from build123d import *

# Parameters (mm, degrees)
CROQUIS1_W              = 471.25
CROQUIS1_H              = 55
SALIENTE_EXTRUIR1_DEPTH = 4
CROQUIS2_W              = 471.25
CROQUIS2_H              = 4
SALIENTE_EXTRUIR2_DEPTH = 55
REDONDEO1_R             = 3
REDONDEO2_R             = 1.5
CORTAR_EXTRUIR1_REACH   = 246.451
CROQUIS3_R              = 2


with BuildPart() as part:
    # Croquis1 → Saliente-Extruir1 (new body)
    with BuildSketch(Plane.XY):
        Rectangle(CROQUIS1_W, CROQUIS1_H)
    extrude(amount=SALIENTE_EXTRUIR1_DEPTH)

    # Croquis2 → Saliente-Extruir2 (add)
    with BuildSketch(Plane(origin=(0, 0, 0), x_dir=(-1, 0, 0), z_dir=(0, 0, -1))):
        with Locations((0, -25.5)):
            Rectangle(CROQUIS2_W, CROQUIS2_H)
    extrude(amount=SALIENTE_EXTRUIR2_DEPTH)

    # Redondeo1
    redondeo1_edges = [part.edges().sort_by_distance(p)[0] for p in [
        (0, -23.5, 0),
    ]]
    fillet(redondeo1_edges, radius=REDONDEO1_R)

    # Redondeo2
    redondeo2_edges = [part.edges().sort_by_distance(p)[0] for p in [
        (0, -27.5, 4),
    ]]
    fillet(redondeo2_edges, radius=REDONDEO2_R)

    # Croquis3 → Cortar-Extruir1 (cut, up to next)
    with BuildSketch(Plane.XY.offset(4), mode=Mode.PRIVATE) as cortar_extruir1_sk1:
        with Locations((-115, -11.2375)):
            Circle(CROQUIS3_R)
    cortar_extruir1_tool1 = extrude(cortar_extruir1_sk1.sketch, amount=-CORTAR_EXTRUIR1_REACH, mode=Mode.PRIVATE) & part.part
    # Croquis3 → Cortar-Extruir1 (cut, up to next)
    with BuildSketch(Plane.XY.offset(4), mode=Mode.PRIVATE) as cortar_extruir1_sk2:
        with Locations((0, -11.2375)):
            Circle(CROQUIS3_R)
    cortar_extruir1_tool2 = extrude(cortar_extruir1_sk2.sketch, amount=-CORTAR_EXTRUIR1_REACH, mode=Mode.PRIVATE) & part.part
    # Croquis3 → Cortar-Extruir1 (cut, up to next)
    with BuildSketch(Plane.XY.offset(4), mode=Mode.PRIVATE) as cortar_extruir1_sk3:
        with Locations((115, -11.2375)):
            Circle(CROQUIS3_R)
    cortar_extruir1_tool3 = extrude(cortar_extruir1_sk3.sketch, amount=-CORTAR_EXTRUIR1_REACH, mode=Mode.PRIVATE) & part.part
    add(cortar_extruir1_tool1.solids().sort_by_distance((-115, -11.2375, 4))[0], mode=Mode.SUBTRACT)
    add(cortar_extruir1_tool2.solids().sort_by_distance((0, -11.2375, 4))[0], mode=Mode.SUBTRACT)
    add(cortar_extruir1_tool3.solids().sort_by_distance((115, -11.2375, 4))[0], mode=Mode.SUBTRACT)


solid = part.part
Could you check a few things on this model? Use its own coordinates, in mm. A direction names the side the tool comes from. Round coordinates to 2 decimals unless told otherwise and drop trailing zeros. Order: outer loops, then holes, each group sorted by start corner. A loop starts at its lowest first (then second) coordinate and runs counter-clockwise, first axis right, second up. Notation, with made-up numbers: M 48,-16.5 L 94,-16.5 A23 ccw 94,17.5 Z; hole C 67,43 d3. An arc over 180 degrees is marked long. One line per item, written item: value.
(1) Imagine slicing it at B-B (y = 21.5). Write out the boundary of the cut face in (x, z) (3 decimals), and give its area (4 significant figures).
Ans:
outline: M -235.625,0 L 235.625,0 L 235.625,4 L -235.625,4 Z
area: 1,885 mm^2
(2) Which directions (+Z, -Z, +X, -X, +Y, -Y) give clear straight access to the entire face, cutting with the end or side of a thin tool? Please do faces 1 (the flat face through (-235.625, -25, -12)), 2 (the flat face through (3, -23.5, -29)).
Ans:
face 1: +Z, -Z, -X, +Y, -Y
face 2: -Z, +X, -X, +Y
(3) Imagine slicing it at C-C (z = -51). Write out the boundary of the cut face in (x, y) (3 decimals), and give its area (4 significant figures).
Ans:
outline: M -235.625,-27.5 L 235.625,-27.5 L 235.625,-23.5 L -235.625,-23.5 Z
area: 1,885 mm^2
(4) I need wall thicknesses on line 1 along Y through (x, z) = (115, 0.8); line 2 along Z through (x, y) = (212.5, -12); line 3 along Y through (x, z) = (151, -50.5). Which ranges of each line are inside material? Lowest first, please. Write a range as from..to.
Ans:
line 1: y = -27.5..-13.24, -9.24..27.5
line 2: z = 0..4
line 3: y = -27.5..-23.5
(5) Imagine slicing it at A-A (x = 153). Write out the boundary of the cut face in (y, z).
Ans:
outline: M -27.5,-55 L -23.5,-55 L -23.5,-3 A3 cw -20.5,0 L 27.5,0 L 27.5,4 L -26,4 A1.5 ccw -27.5,2.5 Z
(6) I'm going to push a flat-ended pin straight in: P1, Ø2.5, axis at x = 115, y = -11.24, coming from the +Z side. Where does the tip first touch, or does it pass through?
Ans:
P1: passes through
